from build123d import *

# Parameters (mm, degrees)
SKETCH1_W           = 106
SKETCH1_H           = 6
SKETCH1_H_2         = 9.4
SKETCH1_H_3         = 8.5
SKETCH1_H_4         = 4.8
BOSS_EXTRUDE4_DEPTH = 4
SKETCH4_W           = 106
SKETCH4_H           = 8.5
CUT_EXTRUDE2_DEPTH  = 3
SKETCH5_W           = 106
SKETCH5_H           = 6
BOSS_EXTRUDE5_DEPTH = 7.6
SKETCH6_R           = 3.5
CUT_EXTRUDE3_DEPTH  = 0.5
SKETCH8_R           = 1
CUT_EXTRUDE4_DEPTH  = 20
SKETCH7_R           = 1
CUT_EXTRUDE5_DEPTH  = 20
SKETCH9_R           = 1
CUT_EXTRUDE6_DEPTH  = 20
SKETCH10_R          = 1.75
CUT_EXTRUDE7_DEPTH  = 20
SKETCH11_R          = 2.9
CUT_EXTRUDE8_DEPTH  = 4.5
CUT_EXTRUDE9_DEPTH  = 3
CUT_EXTRUDE10_DEPTH = 3


with BuildPart() as part:
    # Sketch1 → Boss-Extrude4 (new body)
    with BuildSketch(Plane(origin=(0, 0, 0), x_dir=(1, 0, 0), z_dir=(0, 1, 0))):
        with Locations((53, 20.9)):
            Rectangle(SKETCH1_W, SKETCH1_H)
        with Locations((53, 13.2)):
            Rectangle(SKETCH1_W, SKETCH1_H_2)
        with Locations((53, 4.25)):
            Rectangle(SKETCH1_W, SKETCH1_H_3)
        with Locations((53, -2.4)):
            Rectangle(SKETCH1_W, SKETCH1_H_4)
        with Locations((53, -9.05)):
            Rectangle(SKETCH1_W, SKETCH1_H_3)
        with Locations((53, -18)):
            Rectangle(SKETCH1_W, SKETCH1_H_2)
        with Locations((53, -25.7)):
            Rectangle(SKETCH1_W, SKETCH1_H)
    extrude(amount=BOSS_EXTRUDE4_DEPTH)

    # Sketch4 → Cut-Extrude2 (cut)
    with BuildSketch(Plane(origin=(0, 4, 0), x_dir=(1, 0, 0), z_dir=(0, 1, 0))):
        with Locations((53, 4.25)):
            Rectangle(SKETCH4_W, SKETCH4_H)
        with Locations((53, -9.05)):
            Rectangle(SKETCH4_W, SKETCH4_H)
    extrude(amount=-CUT_EXTRUDE2_DEPTH, mode=Mode.SUBTRACT)

    # Sketch5 → Boss-Extrude5 (add)
    with BuildSketch(Plane(origin=(0, 4, 0), x_dir=(1, 0, 0), z_dir=(0, 1, 0))):
        with Locations((53, 20.9)):
            Rectangle(SKETCH5_W, SKETCH5_H)
        with Locations((53, -25.7)):
            Rectangle(SKETCH5_W, SKETCH5_H)
    extrude(amount=BOSS_EXTRUDE5_DEPTH)

    # Sketch6 → Cut-Extrude3 (cut)
    with BuildSketch(Plane(origin=(0, 1, 0), x_dir=(1, 0, 0), z_dir=(0, 1, 0))):
        with Locations((92, -9.05)):
            Circle(SKETCH6_R)
        with Locations((14, -9.05)):
            Circle(SKETCH6_R)
        with Locations((92, 4.25)):
            Circle(SKETCH6_R)
        with Locations((14, 4.25)):
            Circle(SKETCH6_R)
    extrude(amount=-CUT_EXTRUDE3_DEPTH, mode=Mode.SUBTRACT)

    # Sketch8 → Cut-Extrude4 (cut)
    with BuildSketch(Plane(origin=(0, 0.5, 0), x_dir=(1, 0, 0), z_dir=(0, 1, 0))):
        with Locations((14, 4.25)):
            Circle(SKETCH8_R)
        with Locations((14, -9.05)):
            Circle(SKETCH8_R)
    extrude(amount=-CUT_EXTRUDE4_DEPTH, mode=Mode.SUBTRACT)

    # Sketch7 → Cut-Extrude5 (cut)
    with BuildSketch(Plane(origin=(0, 0.5, 0), x_dir=(1, 0, 0), z_dir=(0, 1, 0))):
        with Locations((92, 4.25)):
            Circle(SKETCH7_R)
    extrude(amount=-CUT_EXTRUDE5_DEPTH, mode=Mode.SUBTRACT)

    # Sketch9 → Cut-Extrude6 (cut)
    with BuildSketch(Plane(origin=(0, 0.5, 0), x_dir=(1, 0, 0), z_dir=(0, 1, 0))):
        with Locations((92, -9.05)):
            Circle(SKETCH9_R)
    extrude(amount=-CUT_EXTRUDE6_DEPTH, mode=Mode.SUBTRACT)

    # Sketch10 → Cut-Extrude7 (cut)
    with BuildSketch(Plane(origin=(0, 11.6, 0), x_dir=(1, 0, 0), z_dir=(0, 1, 0))):
        with Locations((92, 20.9)):
            Circle(SKETCH10_R)
        with Locations((14, 20.9)):
            Circle(SKETCH10_R)
        with Locations((92, -25.7)):
            Circle(SKETCH10_R)
        with Locations((14, -25.7)):
            Circle(SKETCH10_R)
    extrude(amount=-CUT_EXTRUDE7_DEPTH, mode=Mode.SUBTRACT)

    # Sketch11 → Cut-Extrude8 (cut)
    with BuildSketch(Plane(origin=(0, 0, 0), x_dir=(-1, 0, 0), z_dir=(0, -1, 0))):
        with Locations((-92, 20.9)):
            Circle(SKETCH11_R)
        with Locations((-92, -25.7)):
            Circle(SKETCH11_R)
        with Locations((-14, -25.7)):
            Circle(SKETCH11_R)
        with Locations((-14, 20.9)):
            Circle(SKETCH11_R)
    extrude(amount=-CUT_EXTRUDE8_DEPTH, mode=Mode.SUBTRACT)

    # Sketch12 → Cut-Extrude9 (cut)
    with BuildSketch(Plane(origin=(0, 0, -23.9), x_dir=(-1, 0, 0), z_dir=(0, 0, -1))):
        Polygon((-68, 11.6), (-73, 6.6), (-43, 6.6), (-38, 11.6), align=None)
    extrude(amount=-CUT_EXTRUDE9_DEPTH, mode=Mode.SUBTRACT)

    # Sketch13 → Cut-Extrude10 (cut)
    with BuildSketch(Plane.XY.offset(28.7)):
        Polygon((68, 11.6), (73, 6.6), (43, 6.6), (38, 11.6), align=None)
    extrude(amount=-CUT_EXTRUDE10_DEPTH, mode=Mode.SUBTRACT)


solid = part.part
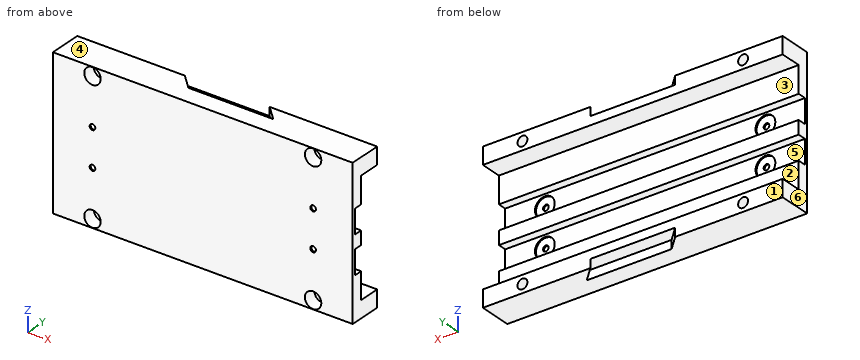
The listing builds one solid part. Answer for the finished solid, in the listing's coordinates (mm). Face numbers are marked on the shaded views. A direction names the side the tool comes from. Give positions to 0.01 mm unless a question says otherwise; leave off trailing zeros. Write each loop counter-clockwise with the first axis right and the second up, starting at its lowest first coordinate (ties: lowest second). Pieces come first, ordered by that corner, then holes. Notation, with made-up numbers: (-10, 73.5) -> (47, 73.5) arc R7 cw to (47, 86.5) -> close; hole circle Ø4 at (5.25, -28). An arc over 180 degrees is marked (long way). Use a Markdown table: item, result.
(1) For the marked faces 1 and 2, determine the directions among +Z, -Z, +X, -X, +Y, -Y from which every point of the face is accessible in a straight line to the end or side of a thin tool.
Return value:
| item | result |
|---|---|
| face 1 | +Z, -Z, +X, -X, +Y |
| face 2 | +X, -X, +Y |
(2) Section B-B, the plane x = 69.5 is taken. Determine the outline of the cut face in (y, z), then the cut area to 3 significant figures.
Return value:
| item | result |
|---|---|
| outline | (0, -23.9) -> (6.6, -23.9) -> (6.6, -20.9) -> (10.1, -20.9) -> (10.1, -23.9) -> (11.6, -23.9) -> (11.6, -17.9) -> (4, -17.9) -> (4, -8.5) -> (1, -8.5) -> (1, 0) -> (4, 0) -> (4, 4.8) -> (1, 4.8) -> (1, 13.3) -> (4, 13.3) -> (4, 22.7) -> (11.6, 22.7) -> (11.6, 28.7) -> (10.1, 28.7) -> (10.1, 25.7) -> (6.6, 25.7) -> (6.6, 28.7) -> (0, 28.7) -> close |
| area | 230 mm2 |
(3) Section C-C, the plane x = 92 is taken. Give the number of separate pieces and of enclosed holes in the cut face, then the cut area to 3 significant figures.
Return value:
| item | result |
|---|---|
| separate pieces | 5 |
| enclosed holes | 0 |
| area | 140 mm2 |
(4) Section D-D, the plane z = -16 is taken. Determine the outline of the cut face in (x, y), then the cut area to 3 significant figures.
Return value:
| item | result |
|---|---|
| outline | (0, 0) -> (106, 0) -> (106, 4) -> (0, 4) -> close |
| area | 424 mm2 |
(5) Find the intervals of material crossed by probe 1 along Z at (x, y) = (73.5, 1.5); probe 2 along Z at (x, y) = (14, 9.75); probe 3 along X at (y, z) = (0.6, -4.25), in increasing order. Write a range as from..to.
Return value:
| item | result |
|---|---|
| probe 1 | -23.9..-8.5, 0..4.8, 13.3..28.7 |
| probe 2 | -23.9..-22.65, -19.15..-17.9, 22.7..23.95, 27.45..28.7 |
| probe 3 | 0..10.5, 17.5..88.5, 95.5..106 |
(6) Determine the mould class of the marked faces 3, 4, 5 and 6 for opening direction Z: released by +Z, released by -Z, zero draft, split by the parting line, or undercut.
Return value:
| item | result |
|---|---|
| face 3 | undercut |
| face 4 | released by +Z |
| face 5 | undercut |
| face 6 | zero draft |
(7) Flat-ended cylindrical pins translate along their axes: P1, Ø4, axis at x = 63.5, y = 9.5, coming from the +Z side; P2, Ø5.5, axis at x = 14, z = 9.05, coming from the +Y side; P3, Ø8, axis at x = 81.5, z = -1, coming from the -Y side; P4, Ø3, axis at x = 49.5, z = 16, coming from the +Y side. Find the tip coordinate at first contact, or state that the pin passes through.
Return value:
| item | result |
|---|---|
| P1 | z = 25.7 |
| P2 | y = 0.5 |
| P3 | y = 0 |
| P4 | y = 4 |
(8) Section A-A, the plane z = 9.05 is taken. Determine the outline of the cut face in (x, y), then the cut area to 3 significant figures.
Return value:
| item | result |
|---|---|
| outline | (0, 0) -> (13, 0) -> (13, 0.5) -> (10.5, 0.5) -> (10.5, 1) -> (0, 1) -> close; (15, 0) -> (91, 0) -> (91, 0.5) -> (88.5, 0.5) -> (88.5, 1) -> (17.5, 1) -> (17.5, 0.5) -> (15, 0.5) -> close; (93, 0) -> (106, 0) -> (106, 1) -> (95.5, 1) -> (95.5, 0.5) -> (93, 0.5) -> close |
| area | 97.0 mm2 |
